Could you check a few things on this model? Use its own coordinates, in mm. Face numbers are marked on the shaded views. A direction names the side the tool comes from. Round coordinates to 2 decimals unless told otherwise and drop trailing zeros. Loops run counter-clockwise (first coordinate to the right, second up) from the corner with the lowest first, then second, coordinate; pieces in that order, holes last. Notation, with made-up numbers: M 41.25,-13.75 L 83.25,-13.75 A25 cw 83.25,8.25 Z; hole C 1,35 d3. An arc over 180 degrees is marked long. Return JSON: item names as keys, results as strings. Group by question number.
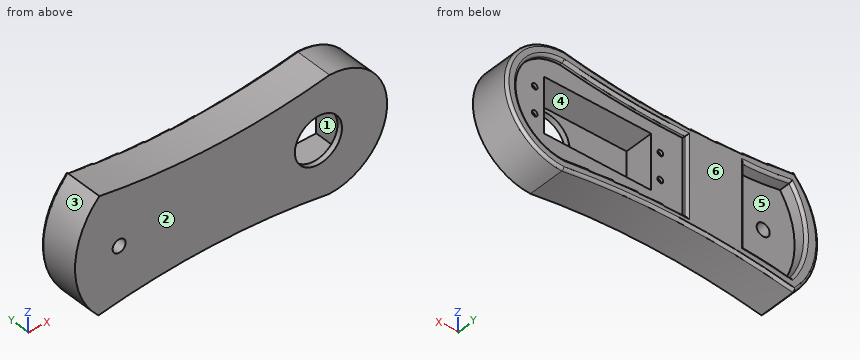
```python
from build123d import *

# Parameters (mm, degrees)
SALIENTE_EXTRUIR1_DEPTH = 15
CORTAR_EXTRUIR2_DEPTH   = 2
CROQUIS3_W              = 41
CROQUIS3_H              = 21
CORTAR_EXTRUIR3_DEPTH   = 11
CROQUIS4_R              = 9
CORTAR_EXTRUIR4_DEPTH   = 101.611139972
CROQUIS5_R              = 1.1
CORTAR_EXTRUIR5_DEPTH   = 1
CORTAR_EXTRUIR13_DEPTH  = 5
CROQUIS7_R              = 2.5
CORTAR_EXTRUIR14_DEPTH  = 101.267649251
REDONDEO2_R             = 1
REDONDEO3_R             = 1


with BuildPart() as part:
    # Croquis1 → Saliente-Extruir1 (new body)
    with BuildSketch(Plane(origin=(0, 0, 0), x_dir=(1, 0, 0), z_dir=(0, 1, 0))):
        with BuildLine():
            ThreePointArc((0, -22), (22, 0), (0, 22))
            ThreePointArc((0, 22), (-44.133753746, 18.164117738), (-88.297835717, 21.633422586))
            ThreePointArc((-88.297835717, 21.633422586), (-97.227552655, -0.44148233), (-87.932501095, -22.365060691))
            ThreePointArc((-87.932501095, -22.365060691), (-43.982219883, -18.335981845), (0, -22))
        make_face()
    extrude(amount=SALIENTE_EXTRUIR1_DEPTH)

    # Croquis2 → Cortar-Extruir2 (cut)
    with BuildSketch(Plane(origin=(0, 15, 0), x_dir=(1, 0, 0), z_dir=(0, 1, 0))):
        with BuildLine():
            Line((-47, 15), (-47, -15))
            ThreePointArc((-47, -15), (-23.432953151, -15.449599362), (0, -18))
            ThreePointArc((0, -18), (18, 0), (0, 18))
            ThreePointArc((0, 18), (-23.433623339, 15.460098979), (-47, 15))
        make_face()
    extrude(amount=-CORTAR_EXTRUIR2_DEPTH, mode=Mode.SUBTRACT)

    # Croquis3 → Cortar-Extruir3 (cut)
    with BuildSketch(Plane(origin=(0, 13, 0), x_dir=(1, 0, 0), z_dir=(0, 1, 0))):
        with Locations((-14.5, 0)):
            Rectangle(CROQUIS3_W, CROQUIS3_H)
    extrude(amount=-CORTAR_EXTRUIR3_DEPTH, mode=Mode.SUBTRACT)

    # Croquis4 → Cortar-Extruir4 (cut, through all)
    with BuildSketch(Plane(origin=(0, 2, 0), x_dir=(1, 0, 0), z_dir=(0, 1, 0))):
        with Locations(Location((-4.25, 0, 0), (0, 0, 270))):
            Circle(CROQUIS4_R)
    extrude(amount=-CORTAR_EXTRUIR4_DEPTH, mode=Mode.SUBTRACT)

    # Croquis5 → Cortar-Extruir5 (cut)
    with BuildSketch(Plane(origin=(0, 13, 0), x_dir=(1, 0, 0), z_dir=(0, 1, 0))):
        with Locations(Location((9.5, 4.9, 0), (0, 0, 270))):
            Circle(CROQUIS5_R)
        with Locations(Location((9.5, -5.1, 0), (0, 0, 270))):
            Circle(CROQUIS5_R)
        with Locations(Location((-38.5, 4.9, 0), (0, 0, 270))):
            Circle(CROQUIS5_R)
        with Locations(Location((-38.5, -5.1, 0), (0, 0, 270))):
            Circle(CROQUIS5_R)
    extrude(amount=-CORTAR_EXTRUIR5_DEPTH, mode=Mode.SUBTRACT)

    # Croquis6 → Cortar-Extruir13 (cut)
    with BuildSketch(Plane(origin=(0, 15, 0), x_dir=(1, 0, 0), z_dir=(0, 1, 0))):
        with BuildLine():
            Line((-68.737734773, 15.427092138), (-68.737734773, -15.97347445))
            ThreePointArc((-68.737734773, -15.97347445), (-77.814777004, -16.578592838), (-86.798496184, -18.010952302))
            ThreePointArc((-86.798496184, -18.010952302), (-92.373186804, -0.406006346), (-86.798496184, 17.198939611))
            ThreePointArc((-86.798496184, 17.198939611), (-77.788079973, 16.109514175), (-68.737734773, 15.427092138))
        make_face()
    extrude(amount=-CORTAR_EXTRUIR13_DEPTH, mode=Mode.SUBTRACT)

    # Croquis7 → Cortar-Extruir14 (cut, through all)
    with BuildSketch(Plane(origin=(0, 10, 0), x_dir=(1, 0, 0), z_dir=(0, 1, 0))):
        with Locations(Location((-80.373306938, 0, 0), (0, 0, 270))):
            Circle(CROQUIS7_R)
    extrude(amount=-CORTAR_EXTRUIR14_DEPTH, mode=Mode.SUBTRACT)

    # Redondeo2
    # the kernel refuses this fillet: 1 mm, written as the material it takes off along each edge
    with BuildSketch(Plane(origin=(-42.931069519, 15, 271.527527752), x_dir=(-0.1874431998722677, 0, -0.9822754434585266), z_dir=(-0.9822754434585266, 0, 0.1874431998722677))) as redondeo2_piece_1:
        with BuildLine():
            CenterArc((253.193727877 + REDONDEO2_R, REDONDEO2_R), REDONDEO2_R, 180, 90)
            Line((253.193727877 + REDONDEO2_R, 0), (253.193727877, 0))
            Line((253.193727877, 0), (253.193727877, REDONDEO2_R))
        make_face()
    revolve(axis=Axis((-42.931069519, 15, 271.527527752), (0, -1, 0)), revolution_arc=21.131483712, mode=Mode.SUBTRACT)
    with BuildSketch(Plane(origin=(0, 15, 0), x_dir=(-0.11357352107267706, 0, 0.9935295945824433), z_dir=(-0.9935295945824433, 0, -0.11357352107267706))) as redondeo2_piece_2:
        with BuildLine():
            CenterArc((22 - REDONDEO2_R, -REDONDEO2_R), REDONDEO2_R, 0, 90)
            Line((22 - REDONDEO2_R, 0), (22, 0))
            Line((22, 0), (22, -REDONDEO2_R))
        make_face()
    revolve(axis=Axis((0, 15, 0), (0, 1, 0)), revolution_arc=193.042709536, mode=Mode.SUBTRACT)
    with BuildSketch(Plane(origin=(-45.249041595, 15, -286.804517852), x_dir=(0.17760158469161672, 0, 0.9841024728731386), z_dir=(0.9841024728731386, 0, -0.17760158469161672))) as redondeo2_piece_3:
        with BuildLine():
            CenterArc((268.642715219 + REDONDEO2_R, REDONDEO2_R), REDONDEO2_R, 180, 90)
            Line((268.642715219, REDONDEO2_R), (268.642715219, 0))
            Line((268.642715219, 0), (268.642715219 + REDONDEO2_R, 0))
        make_face()
    revolve(axis=Axis((-45.249041595, 15, -286.804517852), (0, -1, 0)), revolution_arc=19.984444172, mode=Mode.SUBTRACT)
    with BuildSketch(Plane(origin=(-66.115926768, 15, 0.183151741), x_dir=(-0.6543449081005462, 0, -0.7561962319681894), z_dir=(0.7561962319681894, 0, -0.6543449081005462))) as redondeo2_piece_4:
        with BuildLine():
            CenterArc((31.112698372 - REDONDEO2_R, -REDONDEO2_R), REDONDEO2_R, 0, 90)
            Line((31.112698372 - REDONDEO2_R, 0), (31.112698372, 0))
            Line((31.112698372, 0), (31.112698372, -REDONDEO2_R))
        make_face()
    revolve(axis=Axis((-66.115926768, 15, 0.183151741), (0, 1, 0)), revolution_arc=99.211479347, mode=Mode.SUBTRACT)

    # Redondeo3
    redondeo3_edges = [part.edges().sort_by_distance(p)[0] for p in [
        (-23.433623339, 15, -15.460098979),
        (-47, 15, 0),
        (-23.432953151, 15, 15.449599362),
        (18, 15, 0),
        (-77.788079973, 15, -16.109514175),
        (-68.737734773, 15, 0.273191156),
        (-92.373186804, 15, 0.406006346),
        (-77.814777004, 15, 16.578592838),
    ]]
    fillet(redondeo3_edges, radius=REDONDEO3_R)


solid = part.part
```
1. I'm going to push flat-ended pins straight in: pin 1 Ø3 at (x, z) = (-38.5, 5.1) entering from +Y; pin 2 Ø5.5 at (y, z) = (5.5, -3) entering from -X; pin 3 Ø1.5 at (x, y) = (-12, 9) entering from +Z; pin 4 Ø6 at (x, z) = (-45, 12) entering from -Y. Where does each tip first touch, or does it pass through?
2. I need wall thicknesses on probe 1 along X at (y, z) = (5.5, 0); probe 2 along X at (y, z) = (0.7, 0); probe 3 along X at (y, z) = (12.55, -4.9). Which ranges of each line are inside material? Lowest first, please.
3. If we section it at A-A, the plane y = 8.5: Please give me the cut outline in (x, z), then the cut area to 3 significant figures.
4. On a 3-axis mill with a long thin cutter (end or side, diameter ignored), from which of +Z, -Z, +X, -X, +Y, -Y can I reach the whole of each face in a straight line? I mean the marked faces 1 and 2. Say none if no direction works.
5. If we section it at B-B, the plane z = 0: Give the number of separate pieces and of enclosed holes in the cut face, then the cut area to 3 significant figures.
6. We'd pull the mould along X, two halves only. Please class the marked faces 3, 4, 5 and 6: +X half, -X half, draft (parallel to the pull), parting line (faces both ways), or undercut.
Geometry results:
{
 "1": {"pin 1": "y = 13", "pin 2": "x = -97.23", "pin 3": "z = 20.32", "pin 4": "y = 0"},
 "2": {"probe 1": "-97.23 to -82.87, -77.87 to -35, 6 to 22", "probe 2": "-97.23 to -82.87, -77.87 to -13.25, 4.75 to 22", "probe 3": "-96.81 to -91.91, -68.74 to -39.6, -37.4 to -35, 6 to 8.4, 10.6 to 21.45"},
 "3": {"outline": "M -88.3,-21.63 A268.64 cw 0,-22 A22 ccw 0,22 A253.19 cw -87.93,22.37 A31.11 ccw Z; hole C -80.37,0 d5; hole M -35,-10.5 L 6,-10.5 L 6,10.5 L -35,10.5 Z", "area": "3,590 mm^2"},
 "4": {"face 1": "+Y", "face 2": "+Z, -Z, +X, -X, -Y"},
 "5": {"separate pieces": "3", "enclosed holes": "0", "area": "1,000 mm^2"},
 "6": {"face 3": "-X half", "face 4": "undercut", "face 5": "undercut", "face 6": "draft"}
}
